Verification items for the finished model (mm, model axes). Face numbers are marked on the shaded views. A direction names the side the tool comes from. Coordinates: 2 decimals unless noted, no trailing zeros. Loops run counter-clockwise (first coordinate to the right, second up) from the corner with the lowest first, then second, coordinate; pieces in that order, holes last.
Q1. Sectioned sample at A-A (x = 883.75). Enter the section's corners in (y, z), then the cut area to 3 significant figures.
Q2. Go/stop test with flat-tipped pins: P1, Ø3, axis at y = 3.5, z = 8.5, coming from the -X side; P2, Ø1.9, axis at x = 884.5, z = 3.5, coming from the +Y side; P3, Ø1.5, axis at y = 9, z = 2.5, coming from the +X side. Record where each tip stops, or that it passes through.
Q3. Sectioned sample at C-C (y = 1.5). Enter the section's corners in (x, z), then the cut area to 3 significant figures.
Q4. Access from +Z, -Z, +X, -X, +Y, -Y to the whole of each face (thin tool, end or side, straight path). Record for the marked faces 1, 2, 3 and 4.
Q5. Sectioned sample at B-B (z = 6.25). Enter the section's corners in (x, y).
Q6. Mould release check, pull along X, two halves, no side actions. Record for the marked faces 5, 6, 7 and 8: +X half, -X half, draft (parallel to the pull), parting line (faces both ways), or undercut.
Q7. Sectioned sample at D-D (y = 14.5). Enter the section's corners in (x, z).
Q8. Material ranges on probe 1 along Z at (x, y) = (890.25, -1.5); probe 2 along X at (y, z) = (4.25, 9.75); probe 3 along Y at (x, z) = (884, 8.25), recorded low to high.
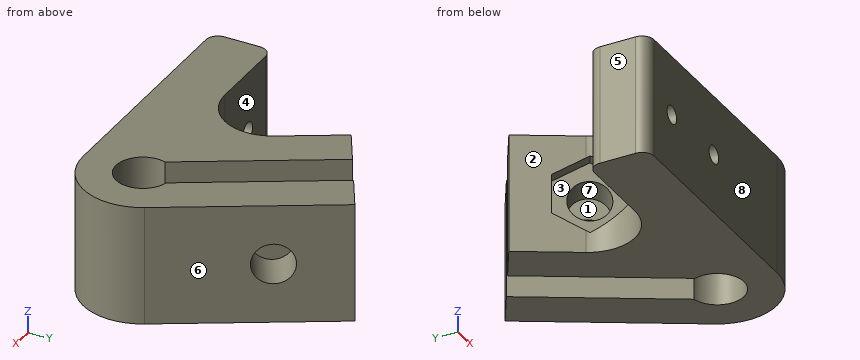
```python
from build123d import *

# Parameters (mm, degrees)
EXTRUDE_1_DEPTH              = 10
CUT_EXTRUDE_1_DEPTH          = 906.195271262
CUT_EXTRUDE_2_REACH          = 458.977
SKETCH_4_W                   = 2.25
SKETCH_4_H                   = 10
HOLE_WIZARD_3_4_3_4_1_D      = 3.4
HOLE_WIZARD_3_4_3_4_1_DEPTH  = 3.5
HOLE_WIZARD_1_5_1_5_1_D      = 1.5
SKETCH_9_W                   = 1.7
SKETCH_9_H                   = 16.290640731
HOLE_WIZARD_1_5_1_5_2_REACH  = 907.297
HOLE_WIZARD_1_5_1_5_2_BORE_R = 0.75
FILLET_1_R                   = 1


with BuildPart() as part:
    # 草图1 → 凸台-拉伸1 (new body)
    with BuildSketch(Plane.XY.offset(10)):
        with BuildLine():
            Line((904.330127019, 2.5), (896.581493223, 15.921027424))
            Line((896.581493223, 15.921027424), (887.921239185, 10.921027424))
            Line((887.921239185, 10.921027424), (890.762395693, 6))
            ThreePointArc((890.762395693, 6), (890.762395693, 2), (887.298294078, 0))
            Line((887.298294078, 0), (880, 0))
            Line((880, 0), (880, -5))
            Line((880, -5), (900, -5))
            ThreePointArc((900, -5), (904.330127019, -2.5), (904.330127019, 2.5))
        make_face()
    extrude(amount=-EXTRUDE_1_DEPTH)

    # 草图2 → 切除-拉伸1 (cut, through all)
    with BuildSketch(Plane(origin=(0, 0, 0), x_dir=(-1, 0, 0), z_dir=(0, 0, -1))):
        with BuildLine():
            Line((-890.952328098, 12.671027424), (-893.55040431, 14.171027424))
            Line((-893.55040431, 14.171027424), (-900.460512614, 2.202368755))
            ThreePointArc((-900.460512614, 2.202368755), (-898.875, 1.948557159), (-897.862436403, 0.702368755))
            Line((-897.862436403, 0.702368755), (-890.952328098, 12.671027424))
        make_face()
    extrude(amount=-CUT_EXTRUDE_1_DEPTH, mode=Mode.SUBTRACT)

    # 草图3 → 切除-拉伸2 (cut, up to next)
    with BuildSketch(Plane(origin=(671.535898385, 387.711431703, 0), x_dir=(-0.4999999999999999, 0.8660254037844386, 0), z_dir=(0.8660254037844387, 0.49999999999999994, 0)), mode=Mode.PRIVATE) as cut_extrude_2_sk1:
        Polygon((-437.644848575, 6.65), (-440.502732408, 8.3), (-443.36061624, 6.65), (-443.36061624, 3.35), (-440.502732408, 1.7), (-437.644848575, 3.35), align=None)
    cut_extrude_2_tool1 = extrude(cut_extrude_2_sk1.sketch, amount=-CUT_EXTRUDE_2_REACH, mode=Mode.PRIVATE) & part.part
    add(cut_extrude_2_tool1.solids().sort_by_distance((891.787265, 6.224875, 5))[0], mode=Mode.SUBTRACT)

    # 草图4 → 切除-旋转1 (revolve, cut)
    with BuildSketch(Plane(origin=(0, 0, 0), x_dir=(1, 0, 0), z_dir=(0, 1, 0))):
        with Locations((901.125, -5)):
            Rectangle(SKETCH_4_W, SKETCH_4_H)
    revolve(axis=Axis((900, 0, 0), (0, 0, 1)), mode=Mode.SUBTRACT)

    # Ø3.4 (3.4) 直径孔1
    with Locations(Plane(origin=(679.330127019, 392.211431703, 0), x_dir=(0, 0, -1), z_dir=(0.8660254037844565, 0.4999999999999692, 0))):
        with Locations((-5, -440.502732408)):
            Hole(HOLE_WIZARD_3_4_3_4_1_D / 2, depth=HOLE_WIZARD_3_4_3_4_1_DEPTH)

    # Ø1.5 (1.5) 直径孔1 (through all)
    with Locations(Plane(origin=(0, 0, 0), x_dir=(1, 0, 0), z_dir=(0, 1, 0))):
        with Locations((883.75, -5)):
            Hole(HOLE_WIZARD_1_5_1_5_1_D / 2)

    # 草图9 → Ø3.4 (3.4) 直径孔2 (revolve, cut)
    with BuildSketch(Plane(origin=(891.787264589, 6.224875001, 5), x_dir=(0.49999999999991085, -0.8660254037844902, 0), z_dir=(0, 0, 1))):
        with Locations((0.85, 8.145320365)):
            Rectangle(SKETCH_9_W, SKETCH_9_H)
    revolve(axis=Axis((886.288003275, 3.049875001, 5), (0.8660254037844902, 0.4999999999999106, 0)), mode=Mode.SUBTRACT)

    # Ø1.5 (1.5) 直径孔2 bore → Ø1.5 (1.5) 直径孔2 (cut, up to next)
    with BuildSketch(Plane(origin=(0, -5, 0), x_dir=(-1, 0, 0), z_dir=(0, -1, 0)), mode=Mode.PRIVATE) as hole_wizard_1_5_1_5_2_sk1:
        with Locations((-890.25, -5)):
            Circle(HOLE_WIZARD_1_5_1_5_2_BORE_R)
    hole_wizard_1_5_1_5_2_tool1 = extrude(hole_wizard_1_5_1_5_2_sk1.sketch, amount=-HOLE_WIZARD_1_5_1_5_2_REACH, mode=Mode.PRIVATE) & part.part
    add(hole_wizard_1_5_1_5_2_tool1.solids().sort_by_distance((890.25, -5, 5))[0], mode=Mode.SUBTRACT)

    # 圆角1
    fillet_1_edges = [part.edges().sort_by_distance(p)[0] for p in [
        (880, -5, 5),
        (880, 0, 5),
    ]]
    fillet(fillet_1_edges, radius=FILLET_1_R)


solid = part.part
```
Geometry check:
1. outline: (-5, 0) - (0, 0) - (0, 4.25) - (-5, 4.25) - close; (-5, 5.75) - (0, 5.75) - (0, 10) - (-5, 10) - close
1. area: 42.5 mm2
2. P1: stops at x = 890.76
2. P2: stops at y = 0
2. P3: stops at x = 901.01
3. outline: (890.42, 0) - (897.4, 0) - (897.4, 10) - (890.42, 10) - (890.42, 5.73) arc R0.75 cw to (890.42, 4.27) - close; (901.68, 0) - (904.77, 0) - (904.77, 10) - (901.68, 10) - close
3. area: 100 mm2
4. face 1: +Z, -Z
4. face 2: +Z, -Z, -X
4. face 3: none
4. face 4: +Z, -Z, -X, +Y
5. outline: (880, -4) arc R1 ccw to (881, -5) - (900, -5) arc R5 ccw to (904.33, 2.5) - (900.16, 9.73) - (897.13, 7.98) - (900.46, 2.2) arc R2.25 cw (long way) to (897.86, 0.7) - (894.53, 6.48) - (892.36, 5.23) - (893.22, 3.75) - (890.99, 2.47) arc R4 cw to (887.3, 0) - (881, 0) arc R1 ccw to (880, -1) - close; (887.92, 10.92) - (889.49, 8.2) - (890.36, 8.7) - (891.21, 7.22) - (893.38, 8.47) - (890.95, 12.67) - close; (893.55, 14.17) - (895.97, 9.97) - (899.01, 11.72) - (896.58, 15.92) - close
6. face 5: -X half
6. face 6: +X half
6. face 7: undercut
6. face 8: draft
7. outline: (894.12, 0) - (897.4, 0) - (897.4, 10) - (894.12, 10) - close
8. probe 1: z = 0 to 4.25, 5.75 to 10
8. probe 2: x = 891.29 to 895.81, 899.28 to 903.32
8. probe 3: y = -5 to 0
